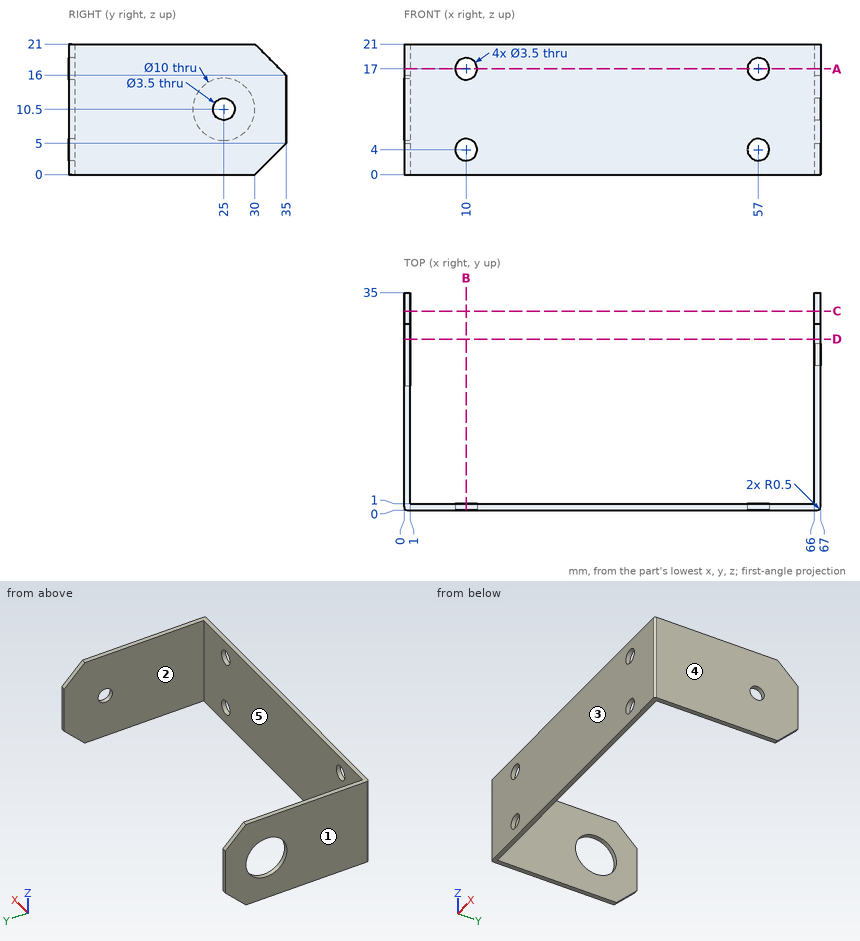
The drawing under review shows one solid part. Ordinate dimensions are in mm from its lowest x, y, z. A direction names the side the tool comes from. Coordinates: 2 decimals unless noted, no trailing zeros. Write each loop counter-clockwise with the first axis right and the second up, starting at its lowest first coordinate (ties: lowest second). Pieces come first, ordered by that corner, then holes. Notation, with made-up numbers: (6, -10.5) - (61, -10.5) arc R14 cw to (61, 6.5) - close; hole circle Ø9 at (58.25, -30.5). An arc over 180 degrees is marked (long way). Answer as CSV lines item,"result".
(1) Tool access review of the marked faces 1 and 2: name each direction out of +Z, -Z, +X, -X, +Y, -Y from which nothing blocks a thin tool from reaching the whole face with its end or side.
Data:
face 1,"+Z, -Z, -X, +Y, -Y"
face 2,"+Z, -Z, +Y"
(2) We need section C-C (y = 32). Give the boundary of the cut face in (x, z), plus the area to 3 significant figures.
Data:
outline,"(0, 2) - (1, 2) - (1, 19) - (0, 19) - close; (66, 2) - (67, 2) - (67, 19) - (66, 19) - close"
area,"34.0 mm2"
(3) We need section D-D (y = 27.5). Give the boundary of the cut face in (x, z).
Data:
outline,"(0, 0) - (1, 0) - (1, 6.17) - (0, 6.17) - close; (0, 14.83) - (1, 14.83) - (1, 21) - (0, 21) - close; (66, 0) - (67, 0) - (67, 21) - (66, 21) - close"
(4) For line 1 along Z through (x, y) = (10, 0.65); line 2 along X through (y, z) = (4, 4); line 3 along Y through (x, z) = (66.3, 10.5), list the stretches that pass through material, from the lowest coordinate up. Write a range as [from, to].
Data:
line 1,"z = [0, 2.25], [5.75, 15.25], [18.75, 21]"
line 2,"x = [0, 1], [66, 67]"
line 3,"y = [0, 23.25], [26.75, 35]"
(5) We need section A-A (z = 17). Give the boundary of the cut face in (x, y).
Data:
outline,"(0, 0.5) arc R0.5 ccw to (0.5, 0) - (8.25, 0) - (8.25, 1) - (1, 1) - (1, 34) - (0, 34) - close; (11.75, 0) - (55.25, 0) - (55.25, 1) - (11.75, 1) - close; (58.75, 0) - (66.5, 0) arc R0.5 ccw to (67, 0.5) - (67, 34) - (66, 34) - (66, 1) - (58.75, 1) - close"
(6) Clearance check with flat-ended pins moving along their axes: pin 1 Ø10 at (x, z) = (53.5, 17.5) entering from +Y; pin 2 Ø3 at (x, z) = (57, 17) entering from -Y; pin 3 Ø6.5 at (y, z) = (26, 11) entering from +X. State where each tip first meets the part, or that it passes through.
Data:
pin 1,"stops at y = 1"
pin 2,"passes through"
pin 3,"stops at x = 67"
(7) Mouldability with a two-part tool opening along X and no side actions: class the marked faces 3, 4 and 5 as pulls with the +X half, pulls with the -X half, needs draft (parallel to the pull), parting line crosses it, or undercut.
Data:
face 3,"needs draft"
face 4,"pulls with the +X half"
face 5,"undercut"
(8) We need section B-B (x = 10). Give the boundary of the cut face in (y, z).
Data:
outline,"(0, 0) - (1, 0) - (1, 2.25) - (0, 2.25) - close; (0, 5.75) - (1, 5.75) - (1, 15.25) - (0, 15.25) - close; (0, 18.75) - (1, 18.75) - (1, 21) - (0, 21) - close"
